Could you check a few things on this model? Use its own coordinates, in mm. Face numbers are marked on the shaded views. A direction names the side the tool comes from. Coordinates: 2 decimals unless noted, no trailing zeros. Loops run counter-clockwise (first coordinate to the right, second up) from the corner with the lowest first, then second, coordinate; pieces in that order, holes last. Notation, with made-up numbers: M 1,60.5 L 45,60.5 A32 cw 45,87.5 Z; hole C 1.25,83.5 d2. An arc over 180 degrees is marked long. Use one line per item in the form item = value. Start each with the question number.
```python
from build123d import *

# Parameters (mm, degrees)
SCHIZZO1_R                   = 3
ESTRUSIONE_ESTRUSIONE1_DEPTH = 15
SCHIZZO2_R                   = 4.95
ESTRUSIONE_ESTRUSIONE2_DEPTH = 8
SMUSSO1_SIZE                 = 0.5
SCHIZZO4_R                   = 2.5
ESTRUSIONE_ESTRUSIONE5_DEPTH = 5
SMUSSO2_SIZE                 = 0.5


with BuildPart() as part:
    # Schizzo1 → Estrusione-Estrusione1 (new body)
    with BuildSketch(Plane(origin=(0, 0, 0), x_dir=(1, 0, 0), z_dir=(0, 1, 0))):
        with Locations(Location((0, 0, 0), (0, 0, 180))):
            Circle(SCHIZZO1_R)
    extrude(amount=-ESTRUSIONE_ESTRUSIONE1_DEPTH)

    # Schizzo2 → Estrusione-Estrusione2 (add)
    with BuildSketch(Plane(origin=(0, 0, 0), x_dir=(1, 0, 0), z_dir=(0, 1, 0))):
        with Locations(Location((0, 0, 0), (0, 0, 180))):
            Circle(SCHIZZO2_R)
    extrude(amount=ESTRUSIONE_ESTRUSIONE2_DEPTH)

    # Smusso1
    smusso1_edges = [part.edges().sort_by_distance(p)[0] for p in [
        (3, -15, 0),
    ]]
    chamfer(smusso1_edges, length=SMUSSO1_SIZE)

    # Schizzo4 → Estrusione-Estrusione5 (add)
    with BuildSketch(Plane(origin=(0, 8, 0), x_dir=(1, 0, 0), z_dir=(0, 1, 0))):
        with Locations(Location((0, 0, 0), (0, 0, 180))):
            Circle(SCHIZZO4_R)
    extrude(amount=ESTRUSIONE_ESTRUSIONE5_DEPTH)

    # Smusso2
    smusso2_edges = [part.edges().sort_by_distance(p)[0] for p in [
        (2.5, 13, 0),
    ]]
    chamfer(smusso2_edges, length=SMUSSO2_SIZE)


solid = part.part
```
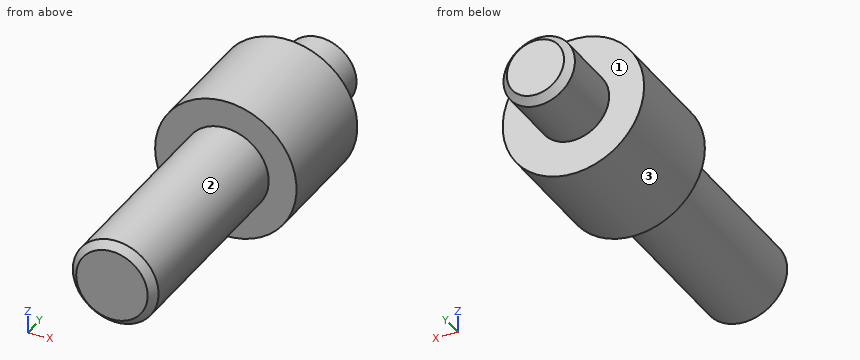
Item 1: Please list where these lines run through material, in increasing order: line 1 along Y through (x, z) = (-4.5, -1.5); line 2 along Z through (x, y) = (0, -4); line 3 along X through (y, z) = (-2, 2.25).
Item 2: I want a section at D-D (y = 3.75). Write out the boundary of the cut face in (x, z).
Item 3: I want a section at A-A (x = 0). Write out the boundary of the cut face in (y, z), plus the area to 3 significant figures.
Item 4: I'm going to push a flat-ended pin straight in: P1, Ø4, axis at x = 1, y = -12, coming from the -Z side. Where does the tip first touch, or does it pass through?
Item 5: I want a section at C-C (y = -12.5). Write out the boundary of the cut face in (x, z), plus the area to 3 significant figures.
Item 6: I want a section at B-B (z = 0). Write out the boundary of the cut face in (x, y), plus the area to 3 significant figures.
Item 7: For the marked faces 1, 2 and 3, which set-ups out of +Z, -Z, +X, -X, +Y, -Y let a thin tool reach every point of the face, with its end or its side?
Worked answers:
q1.line_1 = 0 to 8
q1.line_2 = -3 to 3
q1.line_3 = -1.98 to 1.98
q2.outline = C 0,0 d9.9
q3.outline = M -15,-2.5 L -14.5,-3 L 0,-3 L 0,-4.95 L 8,-4.95 L 8,-2.5 L 12.5,-2.5 L 13,-2 L 13,2 L 12.5,2.5 L 8,2.5 L 8,4.95 L 0,4.95 L 0,3 L -14.5,3 L -15,2.5 Z
q3.area = 194 mm²
q4.P1 = -3
q5.outline = C 0,0 d6
q5.area = 28.3 mm²
q6.outline = M -4.95,0 L -3,0 L -3,-14.5 L -2.5,-15 L 2.5,-15 L 3,-14.5 L 3,0 L 4.95,0 L 4.95,8 L 2.5,8 L 2.5,12.5 L 2,13 L -2,13 L -2.5,12.5 L -2.5,8 L -4.95,8 Z
q6.area = 194 mm²
q7.face_1 = +Y
q7.face_2 = -Y
q7.face_3 = +Y, -Y
